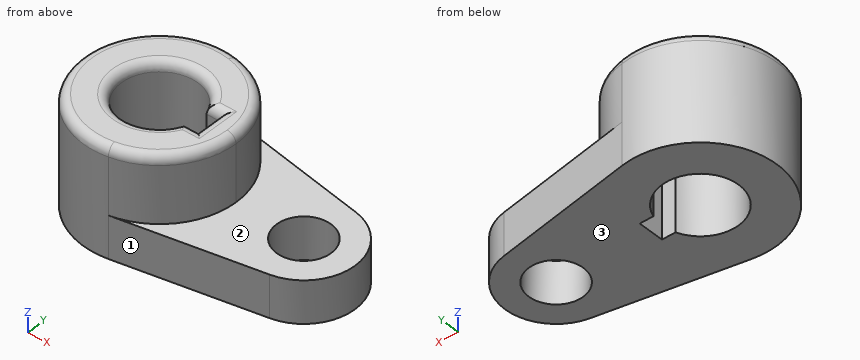
```python
from build123d import *

# Parameters (mm, degrees)
F1_DEPTH = 40.2336
F0_R     = 10.16
F2_DEPTH = 15.7734
F3_R     = 3.302


with BuildPart() as f1:
    # F0 (on Top) → F1 (new body)
    with BuildSketch(Plane.XY):
        with BuildLine():
            ThreePointArc((5.042647, -28.126541), (21.916025, -18.336262), (28.575, 0))
            ThreePointArc((28.575, 0), (21.916025, 18.336262), (5.042647, 28.126541))
            ThreePointArc((5.042647, 28.126541), (-28.575, 0), (5.042647, -28.126541))
        make_face()
        with BuildLine():
            ThreePointArc((13.447765, -4.826), (-14.2875, 0), (13.447765, 4.826))
            Line((13.447765, 4.826), (18.5293, 4.826))
            Line((18.5293, 4.826), (18.5293, -4.826))
            Line((18.5293, -4.826), (13.447765, -4.826))
        make_face(mode=Mode.SUBTRACT)
    extrude(amount=F1_DEPTH)

    # F0 (on Top) → F2 (join)
    with BuildSketch(Plane.XY):
        with BuildLine():
            ThreePointArc((5.042647, -28.126541), (21.916025, -18.336262), (28.575, 0))
            ThreePointArc((28.575, 0), (21.916025, 18.336262), (5.042647, 28.126541))
            ThreePointArc((5.042647, 28.126541), (-28.575, 0), (5.042647, -28.126541))
        make_face()
        with BuildLine():
            ThreePointArc((13.447765, -4.826), (-14.2875, 0), (13.447765, 4.826))
            Line((13.447765, 4.826), (18.5293, 4.826))
            Line((18.5293, 4.826), (18.5293, -4.826))
            Line((18.5293, -4.826), (13.447765, -4.826))
        make_face(mode=Mode.SUBTRACT)
        with BuildLine():
            ThreePointArc((5.042647, 28.126541), (21.916025, 18.336262), (28.575, 0))
            ThreePointArc((28.575, 0), (21.916025, -18.336262), (5.042647, -28.126541))
            Line((5.042647, -28.126541), (57.336765, -18.751028))
            ThreePointArc((57.336765, -18.751028), (73.025, 0), (57.336765, 18.751028))
            Line((57.336765, 18.751028), (5.042647, 28.126541))
        make_face()
        with Locations((53.975, 0)):
            Circle(F0_R, mode=Mode.SUBTRACT)
    extrude(amount=F2_DEPTH)

    # F3
    f3_edges = [f1.edges().sort_by_distance(p)[0] for p in [
        (-5.042647, 28.126541, 40.2336),
        (-14.2875, 0, 40.2336),
        (15.988532, 4.826, 40.2336),
        (18.5293, 0, 40.2336),
        (15.988532, -4.826, 40.2336),
    ]]
    fillet(f3_edges, radius=F3_R)


solid = f1.part
```
The model under review builds one solid part; all positions refer to its coordinate system, in mm. Face numbers are marked on the shaded views. Round coordinates to 2 decimals unless told otherwise and drop trailing zeros. Order: outer loops, then holes, each group sorted by start corner. A loop starts at its lowest first (then second) coordinate and runs counter-clockwise, first axis right, second up. Notation, with made-up numbers: M 57.5,68 L 94.5,68 A12 ccw 94.5,79 Z; hole C -25.75,-36 d11. An arc over 180 degrees is marked long. Use a Markdown table: item, result.
1) Consider section B-B (x = 45.5). Write out the cut boundary in (y, z).
Report:
| item | result |
|---|---|
| outline | M -20.87,0 L -5.6,0 L -5.6,15.77 L -20.87,15.77 Z; M 5.6,0 L 20.87,0 L 20.87,15.77 L 5.6,15.77 Z |
2) Wall thickness on line 1 along X through (y, z) = (-4.5, 14.5); line 2 along Y through (x, z) = (0, 12) (1 decimal); line 3 along X through (y, z) = (-11, 38.5): over which ranges is each line inside the solid? List them lowest first. Write a range as [from, to].
Report:
| item | result |
|---|---|
| line 1 | [-28.22, -13.56], [18.53, 44.87], [63.08, 72.49] |
| line 2 | [-28.6, -14.3], [14.3, 28.6] |
| line 3 | [-25.94, -9.73], [9.73, 25.94] |
3) Insertion check: pin 1 (3 mm diameter, centred on x = -4, z = 27, fed in from +Y); pin 2 (12 mm diameter, centred on y = 17.5, z = 25, fed in from -X); pin 3 (2 mm diameter, centred on y = 20.5, z = 6.5, fed in from -X). Each pin has a flat end and moves straight along its axis. Give the tip position at first contact, or say it passes through.
Report:
| item | result |
|---|---|
| pin 1 | y = 28.47 |
| pin 2 | x = -26.16 |
| pin 3 | x = -20.89 |
4) Draft analysis for pull direction Z (two halves, no side actions). For the marked faces 1, 2 and 3, state which applies: released by +Z, released by -Z, zero draft, split by the parting line, or undercut.
Report:
| item | result |
|---|---|
| face 1 | zero draft |
| face 2 | released by +Z |
| face 3 | released by -Z |
5) Consider section C-C (z = 13). Give the number of separate pieces and of enclosed holes in the cut face, then the cut area to 3 significant figures.
Report:
| item | result |
|---|---|
| separate pieces | 1 |
| enclosed holes | 2 |
| area | 3,450 mm^2 |
6) Consider section D-D (x = 60). Write out the cut boundary in (y, z).
Report:
| item | result |
|---|---|
| outline | M -18.07,0 L -8.18,0 L -8.18,15.77 L -18.07,15.77 Z; M 8.18,0 L 18.07,0 L 18.07,15.77 L 8.18,15.77 Z |
